Read the model definition and answer for the solid it produces. Units are mm, in the model's axes. Coordinates: 2 decimals unless noted, no trailing zeros. Loops run counter-clockwise (first coordinate to the right, second up) from the corner with the lowest first, then second, coordinate; pieces in that order, holes last. Notation, with made-up numbers: (21, -10.5) -> (28, -10.5) arc R14 cw to (28, -4.5) -> close; hole circle Ø1 at (62, 31.5). An arc over 180 degrees is marked (long way). One line per question, with ' | ' between items. Start each with the question number.
```python
from build123d import *

# Parameters (mm, degrees)
SKETCH005_R   = 31.5
SKETCH005_R_2 = 2.5
SKETCH005_R_3 = 1.5
SKETCH005_R_4 = 10
PAD_DEPTH     = 1.5


with BuildPart() as part:
    # Sketch005 → Pad (new body)
    with BuildSketch(Plane.XY.offset(3)):
        Circle(SKETCH005_R)
        with Locations((-10, 25)):
            Circle(SKETCH005_R_2, mode=Mode.SUBTRACT)
        with Locations((10, -25)):
            Circle(SKETCH005_R_2, mode=Mode.SUBTRACT)
        with Locations((-10, -15)):
            Circle(SKETCH005_R_3, mode=Mode.SUBTRACT)
        with Locations((10, 15)):
            Circle(SKETCH005_R_3, mode=Mode.SUBTRACT)
        Circle(SKETCH005_R_4, mode=Mode.SUBTRACT)
    extrude(amount=PAD_DEPTH)


solid = part.part
```
(1) Section D-D on y = 19.5 is taken. Write down the section's boundary in (x, z).
(2) Determine the mould class of faces 1 (the cylindrical face through (-10.33, 27.48, 3.74)), 2 (the flat face through (-7.4, 7.4, 4.5)), 3 (the cylindrical face through (-4.101, 31.232, 3.74)) for opening direction Y: +Y half, -Y half, draft (parallel to the pull), parting line (faces both ways), or undercut.
(3) Section C-C on z = 3.65 is taken. Write down the section's boundary in (x, y), plus the area to 3 significant figures.
(4) Section A-A on y = 0 is taken. Write down the section's boundary in (x, z), plus the area to 3 significant figures.
(5) Find the intervals of material crossed by probe 1 along Y at (x, z) = (-8, 3.2); probe 2 along Y at (x, z) = (0, 3.85); probe 3 along Y at (x, z) = (4.5, 3.85), in increasing order. Write a range as from..to.
(6) Section B-B on x = 4 is taken. Write down the section's boundary in (y, z) (3 decimals).
(7) This flat-tipped pin is pushed along its axis until it touches: pin 1 Ø6.5 at (x, y) = (-10, 25) entering from +Z. Where does it stop, or does it pass through?
Working result:
1) outline: (-24.74, 3) -> (24.74, 3) -> (24.74, 4.5) -> (-24.74, 4.5) -> close
2) face 1: undercut | face 2: draft | face 3: parting line
3) outline: circle Ø63 at (0, 0); hole circle Ø5 at (-10, 25); hole circle Ø3 at (-10, -15); hole circle Ø20 at (0, 0); hole circle Ø5 at (10, -25); hole circle Ø3 at (10, 15) | area: 2,750 mm2
4) outline: (-31.5, 3) -> (-10, 3) -> (-10, 4.5) -> (-31.5, 4.5) -> close; (10, 3) -> (31.5, 3) -> (31.5, 4.5) -> (10, 4.5) -> close | area: 64.5 mm2
5) probe 1: y = -30.47..-6, 6..23.5, 26.5..30.47 | probe 2: y = -31.5..-10, 10..31.5 | probe 3: y = -31.18..-8.93, 8.93..31.18
6) outline: (-31.245, 3) -> (-9.165, 3) -> (-9.165, 4.5) -> (-31.245, 4.5) -> close; (9.165, 3) -> (31.245, 3) -> (31.245, 4.5) -> (9.165, 4.5) -> close
7) pin 1: stops at z = 4.5
